```python
from build123d import *

# Parameters (mm, degrees)
SKETCH1_W           = 56.768800102
SKETCH1_H           = 23.291600102
BOSS_EXTRUDE1_DEPTH = 0.8
CUT_EXTRUDE1_DEPTH  = 1.8
BOSS_EXTRUDE2_DEPTH = 12.065
SKETCH4_R           = 2.413
BOSS_EXTRUDE3_DEPTH = 2.794
SKETCH5_R           = 0.6731
CUT_EXTRUDE2_DEPTH  = 2.794
CUT_EXTRUDE3_DEPTH  = 2.794


with BuildPart() as part:
    # Sketch1 → Boss-Extrude1 (new body)
    with BuildSketch(Plane.XY):
        Rectangle(SKETCH1_W, SKETCH1_H)
    extrude(amount=BOSS_EXTRUDE1_DEPTH)

    # Sketch2 → Cut-Extrude1 (cut, through all)
    with BuildSketch(Plane.XY.offset(0.8)):
        Polygon((-28.384400051, -6.696052583), (-23.434652583, -11.645800051), (-28.384400051, -11.645800051), align=None)
        Polygon((-28.384400051, 6.696052583), (-23.434652583, 11.645800051), (-28.384400051, 11.645800051), align=None)
        Polygon((23.434652583, -11.645800051), (28.384400051, -6.696052583), (28.384400051, -11.645800051), align=None)
        Polygon((23.434652583, 11.645800051), (28.384400051, 6.696052583), (28.384400051, 11.645800051), align=None)
    extrude(amount=-CUT_EXTRUDE1_DEPTH, mode=Mode.SUBTRACT)

    # Sketch3 → Boss-Extrude2 (add)
    with BuildSketch(Plane.XY.offset(0.8)):
        Polygon((23.434652583, 11.645800051), (-23.434652583, 11.645800051), (-28.384400051, 6.696052583), (-28.384400051, -6.696052583), (-23.434652583, -11.645800051), (23.434652583, -11.645800051), (28.384400051, -6.696052583), (28.384400051, 6.696052583), align=None)
        Polygon((-23.103281733, 10.845800051), (-27.584400051, 6.364681733), (-27.584400051, -6.364681733), (-23.103281733, -10.845800051), (23.103281733, -10.845800051), (27.584400051, -6.364681733), (27.584400051, 6.364681733), (23.103281733, 10.845800051), align=None, mode=Mode.SUBTRACT)
    extrude(amount=BOSS_EXTRUDE2_DEPTH)

    # Sketch4 → Boss-Extrude3 (add)
    with BuildSketch(Plane.XY.offset(0.8)):
        with Locations((-21.742400051, 8.813800051)):
            Circle(SKETCH4_R)
        with Locations((18.694400051, -8.686800051)):
            Circle(SKETCH4_R)
    extrude(amount=BOSS_EXTRUDE3_DEPTH)

    # Sketch5 → Cut-Extrude2 (cut)
    with BuildSketch(Plane.XY.offset(3.594)):
        with Locations((-21.742400051, 8.813800051)):
            Circle(SKETCH5_R)
        with Locations((18.694400051, -8.686800051)):
            Circle(SKETCH5_R)
    extrude(amount=-CUT_EXTRUDE2_DEPTH, mode=Mode.SUBTRACT)

    # Sketch6 → Cut-Extrude3 (cut)
    with BuildSketch(Plane(origin=(0, -11.645800051, 0), x_dir=(-1, 0, 0), z_dir=(0, -1, 0))):
        with BuildLine():
            Line((-1.347038418, -12.865), (4.141038418, -12.865))
            Line((4.141038418, -12.865), (2.794, -11.517961582))
            Line((2.794, -11.517961582), (2.794, -2.705))
            ThreePointArc((2.794, -2.705), (1.397, -1.308), (0, -2.705))
            Line((0, -2.705), (0, -11.517961582))
            Line((0, -11.517961582), (-1.347038418, -12.865))
        make_face()
    extrude(amount=-CUT_EXTRUDE3_DEPTH, mode=Mode.SUBTRACT)


solid = part.part
```
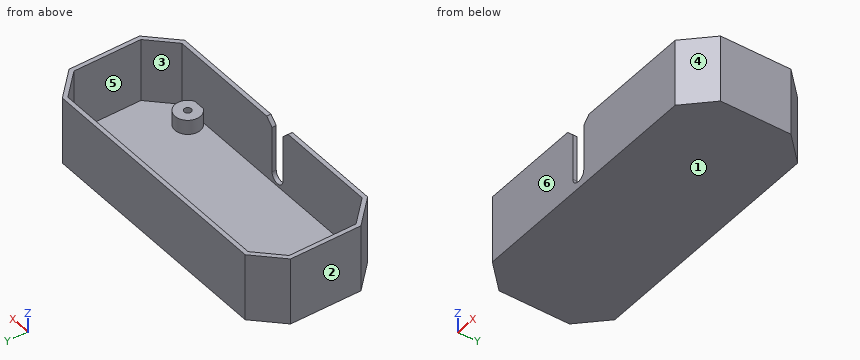
Design review of the part built by this model. Coordinates are the model's own, in mm. Face numbers are marked on the shaded views. A direction names the side the tool comes from. Round coordinates to 2 decimals unless told otherwise and drop trailing zeros. Write each loop counter-clockwise with the first axis right and the second up, starting at its lowest first coordinate (ties: lowest second). Pieces come first, ordered by that corner, then holes.
Item 1: The part is to be moulded in two halves that separate along X. For the marked faces 1, 2, 3 and 4, say which applies: +X half, -X half, draft (parallel to the pull), parting line (faces both ways), or undercut.
Item 2: For the marked faces 5 and 6, list the 3-axis set-ups (+Z, -Z, +X, -X, +Y, -Y) from which the entire face can be reached by the end or side of a thin tool; tool diameter is ignored.
Item 3: Clearance check with flat-ended pins moving along their axes: pin 1 Ø1.1 at (x, y) = (-22, 9) entering from +Z; pin 2 Ø1.5 at (y, z) = (-8.5, 9.5) entering from +X. State where each tip first meets the part, or that it passes through.
Item 4: We need section C-C on y = 2.25. Write out the cut boundary in (x, z) (3 decimals), and give its area (3 significant figures).
Item 5: For probe 1 along Y at (x, z) = (6, 5); probe 2 along X at (y, z) = (-1.25, 7.25); probe 3 along X at (y, z) = (-10, 6.25), list the stretches that pass through material, from the lowest coordinate up.
Item 6: We need section A-A on x = 22. Write out the cut boundary in (y, z) (3 decimals).
Item 7: We need section B-B on z = 2. Write out the cut boundary in (x, y), and give its area (3 significant figures).
Item 8: We need section D-D on z = 7.5. Write out the cut boundary in (x, y).
Returned:
1. face 1: draft
1. face 2: -X half
1. face 3: undercut
1. face 4: +X half
2. face 5: +Z
2. face 6: +Z, -Z, +X, -X, -Y
3. pin 1: stops at z = 3.59
3. pin 2: stops at x = 27.33
4. outline: (-28.384, 0) - (28.384, 0) - (28.384, 12.865) - (27.584, 12.865) - (27.584, 0.8) - (-27.584, 0.8) - (-27.584, 12.865) - (-28.384, 12.865) - close
4. area: 64.7 mm2
5. probe 1: y = -11.65 to -10.85, 10.85 to 11.65
5. probe 2: x = -28.38 to -27.58, 27.58 to 28.38
5. probe 3: x = -25.08 to -23.95, 23.95 to 25.08
6. outline: (-11.646, 0) - (11.646, 0) - (11.646, 12.865) - (10.846, 12.865) - (10.846, 0.8) - (-10.846, 0.8) - (-10.846, 12.865) - (-11.646, 12.865) - close
7. outline: (-28.38, -6.7) - (-23.43, -11.65) - (-2.6, -11.65) - (-2.6, -10.85) - (-23.1, -10.85) - (-27.58, -6.36) - (-27.58, 6.36) - (-23.62, 10.33) arc R2.41 ccw (long way) to (-20.44, 10.85) - (23.1, 10.85) - (27.58, 6.36) - (27.58, -6.36) - (23.1, -10.85) - (19.77, -10.85) arc R2.41 ccw (long way) to (17.62, -10.85) - (-0.19, -10.85) - (-0.19, -11.65) - (23.43, -11.65) - (28.38, -6.7) - (28.38, 6.7) - (23.43, 11.65) - (-23.43, 11.65) - (-28.38, 6.7) - close; hole (-23.26, 10.69) arc R2.41 cw to (-23.04, 10.85) - (-23.1, 10.85) - close; hole circle Ø1.35 at (-21.74, 8.81); hole circle Ø1.35 at (18.69, -8.69)
7. area: 147 mm2
8. outline: (-28.38, -6.7) - (-23.43, -11.65) - (-2.79, -11.65) - (-2.79, -10.85) - (-23.1, -10.85) - (-27.58, -6.36) - (-27.58, 6.36) - (-23.1, 10.85) - (23.1, 10.85) - (27.58, 6.36) - (27.58, -6.36) - (23.1, -10.85) - (0, -10.85) - (0, -11.65) - (23.43, -11.65) - (28.38, -6.7) - (28.38, 6.7) - (23.43, 11.65) - (-23.43, 11.65) - (-28.38, 6.7) - close
